Geometry check sheet. Reference: the model listing, model coordinates, mm. Coordinates: 2 decimals unless noted, no trailing zeros. Write each loop counter-clockwise with the first axis right and the second up, starting at its lowest first coordinate (ties: lowest second). Pieces come first, ordered by that corner, then holes. Notation, with made-up numbers: M -32.75,77.25 L -18.75,77.25 A32 ccw -18.75,107.25 Z; hole C 66.25,-26.75 d6. An arc over 180 degrees is marked long. Put each result on its own line as item: value. Start each with the question number.
1) Cross-section at A-A on y = 0. Record the cut outline in (x, z), plus the area to 3 significant figures.
2) Scan lines: line 1 along X through (y, z) = (-0.1, 38.5); line 2 along Y through (x, z) = (0.6, 36.5); line 3 along Y through (x, z) = (1, 6). Record each from-to range of solid material in increasing order.
3) Cross-section at C-C on z = 1. Record the cut outline in (x, y).
from build123d import *

# Parameters (mm, degrees)
F0_R     = 1.75
F1_DEPTH = 50
F2_R     = 1.75
F3_DEPTH = 7.5
F4_SIZE2 = 7.1153697224
F4_SIZE  = 1
F5_DEPTH = 7.5
F6_SIZE2 = 7.1153697224
F6_SIZE  = 1


with BuildPart() as f1:
    # F0 (on Top) → F1 (new body)
    with BuildSketch(Plane.XY):
        Circle(F0_R)
    extrude(amount=F1_DEPTH)

    # F2 (on face) → F3 (join)
    with BuildSketch(Plane.XY.offset(50)):
        Circle(F2_R)
    extrude(amount=F3_DEPTH)

    # F4
    f4_edges = [f1.edges().sort_by_distance(p)[0] for p in [
        (-1.75, 0, 57.5),
    ]]
    f4_side = f1.faces().sort_by_distance((0, 0, 57.5))[0]
    chamfer(f4_edges, length=F4_SIZE, length2=F4_SIZE2, reference=f4_side)

    # F5 (add): a face of the model
    f5_faces = [f1.faces().sort_by_distance(p)[0] for p in [
        (0, 0, 0),
    ]]
    extrude(f5_faces, amount=F5_DEPTH)

    # F6
    f6_edges = [f1.edges().sort_by_distance(p)[0] for p in [
        (-1.75, 0, -7.5),
    ]]
    f6_side = f1.faces().sort_by_distance((0, 0, -7.5))[0]
    chamfer(f6_edges, length=F6_SIZE, length2=F6_SIZE2, reference=f6_side)


solid = f1.part
Answer key:
1. outline: M -1.75,-0.38 L -0.75,-7.5 L 0.75,-7.5 L 1.75,-0.38 L 1.75,50.38 L 0.75,57.5 L -0.75,57.5 L -1.75,50.38 Z
1. area: 213 mm²
2. line 1: x = -1.75 to 1.75
2. line 2: y = -1.64 to 1.64
2. line 3: y = -1.44 to 1.44
3. outline: C 0,0 d3.5
